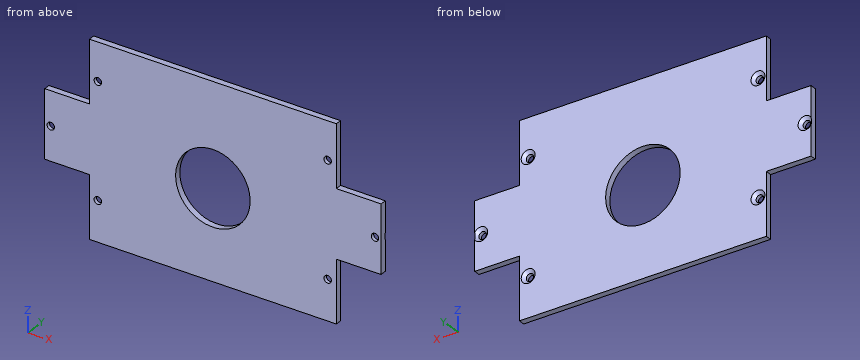
```python
from build123d import *

# Parameters (mm, degrees)
SKETCH1_R                                         = 19.05
BOSS_EXTRUDE1_DEPTH                               = 3.175
CSK_FOR_6_FLAT_HEAD_MACHINE_SCREW_100_D           = 3.7973
CSK_FOR_6_FLAT_HEAD_MACHINE_SCREW_100_CSINK_D     = 7.0866
CSK_FOR_6_FLAT_HEAD_MACHINE_SCREW_100_CSINK_ANGLE = 100
CSK_FOR_6_FLAT_HEAD_MACHINE_SCREW_2_D             = 3.7973
CSK_FOR_6_FLAT_HEAD_MACHINE_SCREW_2_CSINK_D       = 7.0866
CSK_FOR_6_FLAT_HEAD_MACHINE_SCREW_2_CSINK_ANGLE   = 100


with BuildPart() as part:
    # Sketch1 → Boss-Extrude1 (new body)
    with BuildSketch(Plane(origin=(0, 0, 0), x_dir=(1, 0, 0), z_dir=(0, 1, 0))):
        Polygon((-63.899577335, 57.690677645), (62.306672665, 57.690677645), (62.306672665, 25.940677645), (85.166672665, 25.940677645), (85.166672665, -8.603322355), (62.306672665, -8.603322355), (62.306672665, -40.353322355), (-63.899577335, -40.353322355), (-63.899577335, -8.603322355), (-86.759577335, -8.603322355), (-86.759577335, 25.940677645), (-63.899577335, 25.940677645), align=None)
        with Locations(Location((-0.796452335, 11.970677645, 0), (0, 0, 270))):
            Circle(SKETCH1_R, mode=Mode.SUBTRACT)
    extrude(amount=BOSS_EXTRUDE1_DEPTH)

    # CSK for _6 Flat Head Machine Screw _100 (through all)
    with Locations(Plane(origin=(0, 3.175, 0), x_dir=(1, 0, 0), z_dir=(0, 1, 0))):
        with Locations((-59.613327335, 37.246553163), (-59.613327335, -21.054053163), (57.861672665, -21.054053163), (57.861672665, 37.246553163)):
            CounterSinkHole(CSK_FOR_6_FLAT_HEAD_MACHINE_SCREW_100_D / 2, CSK_FOR_6_FLAT_HEAD_MACHINE_SCREW_100_CSINK_D / 2, counter_sink_angle=CSK_FOR_6_FLAT_HEAD_MACHINE_SCREW_100_CSINK_ANGLE)

    # CSK for _6 Flat Head Machine Screw _ 2 (through all)
    with Locations(Plane(origin=(0, 3.175, 0), x_dir=(1, 0, 0), z_dir=(0, 1, 0))):
        with Locations((82.071047665, 8.73125), (-83.663952335, 8.73125)):
            CounterSinkHole(CSK_FOR_6_FLAT_HEAD_MACHINE_SCREW_2_D / 2, CSK_FOR_6_FLAT_HEAD_MACHINE_SCREW_2_CSINK_D / 2, counter_sink_angle=CSK_FOR_6_FLAT_HEAD_MACHINE_SCREW_2_CSINK_ANGLE)


solid = part.part
```
Input: part model. Units: mm. Frame: model coordinates. Coordinates: 2 decimals unless noted, no trailing zeros. Write each loop counter-clockwise with the first axis right and the second up, starting at its lowest first coordinate (ties: lowest second). Pieces come first, ordered by that corner, then holes.
1) Material intervals for line 1 along X through (y, z) = (1.4, -8); line 2 along X through (y, z) = (1.35, 17.5); line 3 along Z through (x, y) = (-69.5, 2.9), sorted ascending.
2) Section A-A on x = 15. Output: boundary loops of the cut face in (y, z) (3 decimals), and give its area (3 significant figures).
3) Pin query (flat end, axial travel): pin 1 Ø1 at (y, z) = (2, 27.5) entering from +X; pin 2 Ø1 at (x, y) = (71.5, 1) entering from +Z; pin 3 Ø5 at (x, z) = (-59.61, 21.05) entering from +Y; pin 4 Ø3 at (x, z) = (57.86, 21.05) entering from +Y. Return the tip coordinate at first contact, or that it passes through.
4) Section B-B on z = -1. Output: boundary loops of the cut face in (x, y) (3 decimals), and give its area (3 significant figures).
5) Section C-C on x = -73.5. Output: boundary loops of the cut face in (y, z) (3 decimals).
6) Section D-D on z = -43.5. Output: boundary loops of the cut face in (x, y) (3 decimals).
Check result:
1. line 1: x = -86.76 to -85.42, -81.91 to -19.43, 17.84 to 80.32, 83.82 to 85.17
1. line 2: x = -63.9 to 62.31
1. line 3: z = -25.94 to 8.6
2. outline: (0, -57.691) - (3.175, -57.691) - (3.175, -22.618) - (0, -22.618) - close; (0, -1.323) - (3.175, -1.323) - (3.175, 40.353) - (0, 40.353) - close
2. area: 244 mm2
3. pin 1: stops at x = 62.31
3. pin 2: stops at z = 8.6
3. pin 3: stops at y = 2.3
3. pin 4: passes through
4. outline: (-86.76, 0) - (-16.37, 0) - (-16.37, 3.175) - (-86.76, 3.175) - close; (14.777, 0) - (85.167, 0) - (85.167, 3.175) - (14.777, 3.175) - close
4. area: 447 mm2
5. outline: (0, -25.941) - (3.175, -25.941) - (3.175, 8.603) - (0, 8.603) - close
6. outline: (-63.9, 0) - (62.307, 0) - (62.307, 3.175) - (-63.9, 3.175) - close
